from build123d import *

# Parameters (mm, degrees)
F0_W      = 70
F0_H      = 135
F1_DEPTH  = 10
F2_T      = -2.5
F3_R      = 5
F4_R      = 5
F5_R      = 5
F6_R      = 5
F7_W      = 1
F7_H      = 4
F8_DEPTH  = 1
F9_DEPTH  = 2
F11_DEPTH = 1


with BuildPart() as f1:
    # F0 (on Top) → F1 (new body)
    with BuildSketch(Plane.XY):
        Rectangle(F0_W, F0_H)
    extrude(amount=F1_DEPTH)

    # F2
    f2_openings = [f1.faces().sort_by_distance(p)[0] for p in [
        (0, 0, 0),
    ]]
    offset(amount=F2_T, openings=f2_openings)

    # F3
    f3_edges = [f1.edges().sort_by_distance(p)[0] for p in [
        (0, 67.5, 10),
        (35, 0, 10),
        (35, 67.5, 5),
    ]]
    fillet(f3_edges, radius=F3_R)

    # F4
    f4_edges = [f1.edges().sort_by_distance(p)[0] for p in [
        (33.535534, -67.5, 8.535534),
        (-2.5, -67.5, 10),
    ]]
    fillet(f4_edges, radius=F4_R)

    # F5
    f5_edges = [f1.edges().sort_by_distance(p)[0] for p in [
        (-35, 0, 10),
        (-35, -66.035534, 8.535534),
    ]]
    fillet(f5_edges, radius=F5_R)

    # F6
    f6_edges = [f1.edges().sort_by_distance(p)[0] for p in [
        (32.5, 65, 3.75),
        (-32.5, 65, 3.75),
        (32.5, -65, 3.75),
        (-32.5, -65, 3.75),
    ]]
    fillet(f6_edges, radius=F6_R)

    # F7 (on face) → F8 (join)
    with BuildSketch(Plane(origin=(0, 0, 0), x_dir=(1, 0, 0), z_dir=(0, 0, -1))):
        with Locations((-33.75, 0)):
            Rectangle(F7_W, F7_H)
        with Locations((33.75, 0)):
            Rectangle(F7_W, F7_H)
    extrude(amount=F8_DEPTH)

    # F9 (cut): a face of the model
    f9_faces = [f1.faces().sort_by_distance(p)[0] for p in [
        (0, 0, 10),
    ]]
    extrude(f9_faces, amount=-F9_DEPTH, mode=Mode.SUBTRACT)

    # F10 (on face) → F11 (cut)
    with BuildSketch(Plane.XY.offset(8)):
        with BuildLine():
            Line((5, 57.5), (0, 57.5))
            Line((0, 57.5), (-4.9842596054, 57.5))
            ThreePointArc((-4.9842596054, 57.5), (-6.4842596054, 56), (-4.9842596054, 54.5))
            Line((-4.9842596054, 54.5), (5.0273956731, 54.5))
            ThreePointArc((5.0273956731, 54.5), (6.5000625423, 56.0135733205), (5, 57.5))
        make_face()
    extrude(amount=-F11_DEPTH, mode=Mode.SUBTRACT)


solid = f1.part
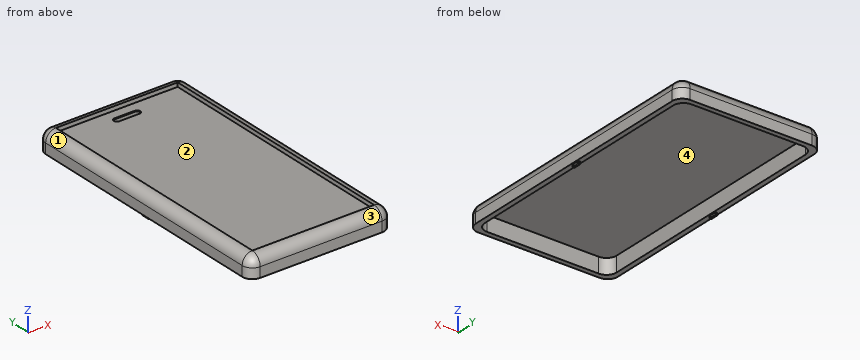
Could you check a few things on this model? Use its own coordinates, in mm. Face numbers are marked on the shaded views. Coordinates: 2 decimals unless noted, no trailing zeros. Order: outer loops, then holes, each group sorted by start corner. A loop starts at its lowest first (then second) coordinate and runs counter-clockwise, first axis right, second up. Notation, with made-up numbers: (8, 82) -> (51, 82) arc R34 cw to (51, 112) -> close; hole circle Ø11 at (50, 87). An arc over 180 degrees is marked (long way). One line per question, with ' | ' between items.
Q1. Imagine slicing it at B-B on x = 26. Please give me the cut outline in (y, z), and give its area (3 significant figures).
Return value:
outline: (-67.5, 0) -> (-65, 0) -> (-65, 7.5) -> (65, 7.5) -> (65, 0) -> (67.5, 0) -> (67.5, 5) arc R5 ccw to (62.5, 10) -> (62.5, 8) -> (-62.5, 8) -> (-62.5, 10) arc R5 ccw to (-67.5, 5) -> close | area: 114 mm²
Q2. If I drill on L1, parallel to X at y = 5, z = 0.25; L2, parallel to Y at x = 13, z = 1.75; L3, parallel to Y at x = 30, z = 4.5, over which ranges is the centre line in solid material (lowest first)?
Return value:
L1: -35 to -32.5, 32.5 to 35 | L2: -67.5 to -65, 65 to 67.5 | L3: -67.5 to -64.33, 64.33 to 67.5
Q3. I'm going to push flat-ended pins straight in: P1, Ø0.5, axis at y = -1, z = -0.5, coming from the -X side; P2, Ø8, axis at x = -14.5, y = -15.5, coming from the +Z side; P3, Ø1.6, axis at y = 30, z = 9.5, coming from the -X side. Where does each tip first touch, or does it pass through?
Return value:
P1: x = -34.25 | P2: z = 8 | P3: x = -33.36
Q4. Thinking about a two-plate mould opening in X: for the marked faces 1, 2, 3 and 4, which applies, pulls with the +X half, pulls with the -X half, needs draft (parallel to the pull), parting line crosses it, or undercut?
Return value:
face 1: pulls with the -X half | face 2: undercut | face 3: needs draft | face 4: undercut
Q5. Imagine slicing it at A-A on y = 56. Please give me the cut outline in (x, z).
Return value:
outline: (-35, 0) -> (-32.5, 0) -> (-32.5, 7.5) -> (-6.48, 7.5) -> (-6.48, 8) -> (-30, 8) -> (-30, 10) arc R5 ccw to (-35, 5) -> close; (6.5, 7.5) -> (32.5, 7.5) -> (32.5, 0) -> (35, 0) -> (35, 5) arc R5 ccw to (30, 10) -> (30, 8) -> (6.5, 8) -> close
